Here's how the part is built. I have some questions about the finished solid (model axes, mm). Face numbers are marked on the shaded views. A direction names the side the tool comes from. Coordinates: 2 decimals unless noted, no trailing zeros. Write each loop counter-clockwise with the first axis right and the second up, starting at its lowest first coordinate (ties: lowest second). Pieces come first, ordered by that corner, then holes. Notation, with made-up numbers: (71, 7.5) -> (78, 7.5) arc R28 ccw to (78, 45.5) -> close; hole circle Ø4 at (-22.5, 45). An arc over 180 degrees is marked (long way). Put each result on its own line as item: value. Start each with the question number.
Item 1: I want a section at B-B, the plane x = -6. List the corners of the cut face in (y, z) for me.
Item 2: If we mould it in two halves opening along Y, with no side actions, what happens to the marked faces 5, 6, 7 and 8? For each: released by +Y, released by -Y, zero draft, split by the parting line, or undercut.
Item 3: I need wall thicknesses on line 1 (Z direction, x = -11.7, y = 0); line 2 (X direction, y = -3.25, z = 2.25); line 3 (X direction, y = 0.5, z = 7.75). Which ranges of each line are inside material? Lowest first, please. Write a range as [from, to].
Item 4: On a 3-axis mill with a long thin cutter (end or side, diameter ignored), from which of +Z, -Z, +X, -X, +Y, -Y can I reach the whole of each face in a straight line? I mean the marked faces 1, 2, 3 and 4. Say none if no direction works.
Item 5: I want a section at A-A, the plane x = -9.75. List the corners of the cut face in (y, z) for me (3 decimals).
Item 6: For pin 1 (4 mm diameter, centred on y = 0, z = 5, fed in from -X); pin 2 (1.1 mm diameter, centred on x = 4, z = 5.5, fed in from +Y) (3 decimals); pin 3 (2 mm diameter, centred on y = 4, z = 4.5, fed in from +X), each with a flat end and sliding along its axis, tell me the tip position at first contact or that it passes through.
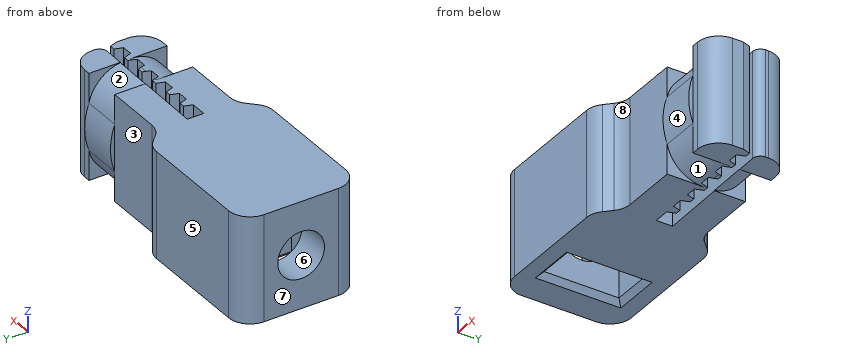
from build123d import *

# Parameters (mm, degrees)
PAD002_DEPTH    = 3.7
PAD001_DEPTH    = 3.5
PAD_DEPTH       = 10
SKETCH001_R     = 2.2
POCKET_DEPTH    = 13.5
CHAMFER_SIZE    = 0.5
FILLET_R        = 2
FILLET001_R     = 0.75
SKETCH004_W     = 3.7
SKETCH004_H     = 4.441354
PAD003_DEPTH    = 2
POCKET001_DEPTH = 3.7
SKETCH006_W     = 3.7
SKETCH006_H     = 4.441354
PAD004_DEPTH    = 2
POCKET002_DEPTH = 3.7


with BuildPart() as pad002:
    # Sketch003 → Pad002 (new body)
    with BuildSketch(Plane.YZ.offset(11.1)):
        with BuildLine():
            Line((-1.31066, 11.5), (1.31066, 11.5))
            ThreePointArc((5.25, 7.56066), (4.096194, 10.346194), (1.31066, 11.5))
            Line((5.25, 7.56066), (5.25, 2.43934))
            ThreePointArc((1.31066, -1.5), (4.096194, -0.346194), (5.25, 2.43934))
            Line((1.31066, -1.5), (-1.31066, -1.5))
            ThreePointArc((-5.25, 2.43934), (-4.096194, -0.346194), (-1.31066, -1.5))
            Line((-5.25, 2.43934), (-5.25, 7.56066))
            ThreePointArc((-1.31066, 11.5), (-4.096194, 10.346194), (-5.25, 7.56066))
        make_face()
        with BuildLine():
            Line((-0.25, 10), (0.25, 10))
            ThreePointArc((3.75, 6.5), (2.724874, 8.974874), (0.25, 10))
            Line((3.75, 6.5), (3.75, 3.5))
            ThreePointArc((0.25, 0), (2.724874, 1.025126), (3.75, 3.5))
            Line((0.25, 0), (-0.25, 0))
            ThreePointArc((-3.75, 3.5), (-2.724874, 1.025126), (-0.25, 0))
            Line((-3.75, 3.5), (-3.75, 6.5))
            ThreePointArc((-0.25, 10), (-2.724874, 8.974874), (-3.75, 6.5))
        make_face(mode=Mode.SUBTRACT)
    extrude(amount=-PAD002_DEPTH)


with BuildPart() as pad001:
    # Sketch002 → Pad001 (new body)
    with BuildSketch(Plane.YZ.offset(-7)):
        Polygon((3.525, 2.96484), (3.525, 7.03516), (0, 9.070319), (-3.525, 7.03516), (-3.525, 2.96484), (-3.525, 0), (3.525, 0), align=None)
    extrude(amount=-PAD001_DEPTH)


with BuildPart() as pocket002:
    # Sketch → Pad (new body)
    with BuildSketch(Plane.XY):
        Polygon((2.75, -0.675), (3, 0.075), (3.5, 0.075), (3.75, -0.675), (4.75, -0.675), (5, 0.075), (5.5, 0.075), (5.75, -0.675), (6.75, -0.675), (7, 0.075), (7.5, 0.075), (7.75, -0.675), (8.75, -0.675), (9, 0.075), (9.5, 0.075), (9.75, -0.675), (10.75, -0.675), (11, 0.075), (11.5, 0.075), (11.75, -0.675), (12.75, -0.675), (13, 0.075), (13.5, 0.075), (13.75, -0.675), (13.75, -3.675), (1.25, -3.675), (-0.575, -5.5), (-13.75, -5.5), (-13.75, 5.5), (-0.575, 5.5), (1.25, 3.675), (13.75, 3.675), (13.75, 0.675), (1.25, 0.875), (1.25, -0.675), align=None)
    extrude(amount=PAD_DEPTH)

    # Sketch001 → Pocket (cut)
    with BuildSketch(Plane(origin=(-13.75, 0, 0), x_dir=(0, -1, 0), z_dir=(-1, 0, 0))):
        with Locations((0, 5)):
            Circle(SKETCH001_R)
    extrude(amount=-POCKET_DEPTH, mode=Mode.SUBTRACT)

    # Cut: cut Pad001
    add(pad001.part, mode=Mode.SUBTRACT)

    # Cut001: cut Pad002
    add(pad002.part, mode=Mode.SUBTRACT)

    # Chamfer
    chamfer_edges = [pocket002.edges().sort_by_distance(p)[0] for p in [
        (-7, 0, 0),
        (-8.75, -3.525, 0),
        (-10.5, 0, 0),
        (-8.75, 3.525, 0),
    ]]
    chamfer(chamfer_edges, length=CHAMFER_SIZE)

    # Fillet
    fillet_edges = [pocket002.edges().sort_by_distance(p)[0] for p in [
        (13.75, 3.675, 5),
        (1.25, 3.675, 5),
        (-0.575, 5.5, 5),
        (-13.75, 5.5, 5),
        (13.75, -3.675, 5),
        (1.25, -3.675, 5),
        (-0.575, -5.5, 5),
        (-13.75, -5.5, 5),
    ]]
    fillet(fillet_edges, radius=FILLET_R)

    # Fillet001
    fillet001_edges = [pocket002.edges().sort_by_distance(p)[0] for p in [
        (13.75, 0.675, 5),
    ]]
    fillet(fillet001_edges, radius=FILLET001_R)

    # Sketch004 → Pad003 (new body)
    with BuildSketch(Plane.XZ.offset(3.675)):
        with Locations((9.25, 5)):
            Rectangle(SKETCH004_W, SKETCH004_H)
    extrude(amount=PAD003_DEPTH)

    # Sketch005 → Pocket001 (cut)
    with BuildSketch(Plane.YZ.offset(11.1)):
        with BuildLine():
            ThreePointArc((-3.675, 7.220677), (-4.075959, 5), (-3.675, 2.779323))
            Line((-3.675, 2.779323), (-5.675, 2.779323))
            Line((-5.675, 2.779323), (-5.675, 7.220677))
            Line((-5.675, 7.220677), (-3.675, 7.220677))
        make_face()
    extrude(amount=-POCKET001_DEPTH, mode=Mode.SUBTRACT)

    # Sketch006 → Pad004 (new body)
    with BuildSketch(Plane(origin=(0, 3.675, 0), x_dir=(-1, 0, 0), z_dir=(0, 1, 0))):
        with Locations((-9.25, 5)):
            Rectangle(SKETCH006_W, SKETCH006_H)
    extrude(amount=PAD004_DEPTH)

    # Sketch007 → Pocket002 (cut)
    with BuildSketch(Plane.YZ.offset(11.1)):
        with BuildLine():
            ThreePointArc((3.675, 2.779323), (4.075959, 5), (3.675, 7.220677))
            Line((3.675, 7.220677), (5.675, 7.220677))
            Line((5.675, 7.220677), (5.675, 2.779323))
            Line((5.675, 2.779323), (3.675, 2.779323))
        make_face()
    extrude(amount=-POCKET002_DEPTH, mode=Mode.SUBTRACT)


solid = pocket002.part
Calculated:
1. outline: (-5.5, 0) -> (5.5, 0) -> (5.5, 10) -> (-5.5, 10) -> close; hole circle Ø4.4 at (0, 5)
2. face 5: released by +Y
2. face 6: undercut
2. face 7: zero draft
2. face 8: released by -Y
3. line 1: z = [0, 2.8], [7.2, 10]
3. line 2: x = [-13.75, -10.5], [-7, 12.98]
3. line 3: x = [-13.75, -10.5], [-7, 1.25]
4. face 1: -Z, -Y
4. face 2: +Z, +Y
4. face 3: +Z, -Z, +Y
4. face 4: +X, -Y
5. outline: (-5.5, 0) -> (-4.025, 0) -> (-3.525, 0.5) -> (-3.525, 7.035) -> (0, 9.07) -> (3.525, 7.035) -> (3.525, 0.5) -> (4.025, 0) -> (5.5, 0) -> (5.5, 10) -> (-5.5, 10) -> close
6. pin 1: stops at x = -0.25
6. pin 2: stops at y = 3.675
6. pin 3: stops at x = 13.25
